Part model, mm, in its own coordinate system. A direction names the side the tool comes from. Coordinates: 2 decimals unless noted, no trailing zeros. Write each loop counter-clockwise with the first axis right and the second up, starting at its lowest first coordinate (ties: lowest second). Pieces come first, ordered by that corner, then holes. Notation, with made-up numbers: M 26.25,46.5 L 30.25,46.5 A25 cw 30.25,82.5 Z; hole C 61.5,72.25 d7. An arc over 180 degrees is marked long. Use a Markdown table: item, result. Add a question column.
Q1. Slice it at B-B on y = 94. Write the cut outline in (x, z).
Q2. Mould opens along X. For faces 1 (the flat face through (-31.2, 107.95, 11.5)), 2 (the cylindrical face through (-8.21, 1.25, -26.07)), 3 (the cylindrical face through (-11.437, 103.567, -36.316)) say: released by +X, released by -X, zero draft, split by the parting line, or undercut.
Q3. Pin check, flat tips, straight feed: pin 1 Ø5 at (y, z) = (94.5, -28.5) entering from -X; pin 2 Ø4 at (x, z) = (29, 27.5) entering from -Y; pin 3 Ø4 at (x, y) = (-28, 39.5) entering from -Z. Stop position of each tip, or through.
Q4. Slice it at A-A on y = 20. Write the cut outline in (x, z).
Q5. Tool access for faces 4 (the flat face through (-24, 0, -14)), 5 (the flat face through (-26, 2.54, 9)), 6 (the flat face through (20, 99.06, 31)): list every direction of +Z, -Z, +X, -X, +Y, -Y with a clear straight run to the whole face (end or side of a thin tool).
Q6. Wall check: L1, parallel to X at y = 106.75, z = 0; L2, parallel to X at y = 0.7, z = 0; L3, parallel to Z at x = -22, y = 80. Give the ranges that are in metal, low to high. Write a range as from..to.
from build123d import *

# Parameters (mm, degrees)
CUT_EXTRUDE2_DEPTH = 45.212
CIRPATTERN2_COUNT  = 4


with BuildPart() as part:
    # Sketch2 → Revolve2 (revolve)
    with BuildSketch(Plane.XY, mode=Mode.PRIVATE) as revolve2_sk:
        Polygon((27.3304, 2.54), (27.3304, 0), (31.623, 0), (36.4998, 99.06), (38.0746, 99.06), (38.0746, 107.95), (32.9946, 107.95), (32.9946, 102.87), (29.083, 2.54), align=None)
    revolve(revolve2_sk.sketch.rotate(Axis((0, 0, 0), (0, 1, 0)), 90), axis=Axis((0, 0, 0), (0, 1, 0)))

    # Sketch5 → Cut-Extrude2 (cut)
    with BuildSketch(Plane.XY):
        with BuildLine():
            ThreePointArc((3.175, 103.505), (2.24506403, 105.75006403), (0, 106.68))
            Line((0, 106.68), (0, 100.33))
            ThreePointArc((0, 100.33), (2.24506403, 101.25993597), (3.175, 103.505))
        make_face()
        with BuildLine():
            Line((0, 100.33), (0, 106.68))
            ThreePointArc((0, 106.68), (-3.175, 103.505), (0, 100.33))
        make_face()
    cut_extrude2 = extrude(amount=-CUT_EXTRUDE2_DEPTH, mode=Mode.SUBTRACT)

    # CirPattern2: Cut-Extrude2 ×4 about axis
    cirpattern2_axis = Axis((0, 0, 0), (0, -1, 0))
    for i in range(1, CIRPATTERN2_COUNT):
        add(cut_extrude2.rotate(cirpattern2_axis, i * 360 / CIRPATTERN2_COUNT), mode=Mode.SUBTRACT)


solid = part.part
Recorded:
| question | item | result |
|---|---|---|
| 1 | outline | C 0,0 d72.5; hole C 0,0 d65.3 |
| 2 | face 1 | zero draft |
| 2 | face 2 | undercut |
| 2 | face 3 | split by the parting line |
| 3 | pin 1 | x = -25.3 |
| 3 | pin 2 | y = 99.06 |
| 3 | pin 3 | z = -21.24 |
| 4 | outline | C 0,0 d65.22; hole C 0,0 d59.53 |
| 5 | face 4 | +Z, -Z, +X, -X, -Y |
| 5 | face 5 | +Y |
| 5 | face 6 | -Y |
| 6 | L1 | -38.07..-32.99, 32.99..38.07 |
| 6 | L2 | -31.66..-27.33, 27.33..31.66 |
| 6 | L3 | -27.94..-23.38, 23.38..27.94 |
